```python
from build123d import *

# Parameters (mm, degrees)
SKETCH_1_W           = 58
SKETCH_1_H           = 13
EXTRUDE_1_DEPTH      = 6
SKETCH_9_W           = 58
SKETCH_9_H           = 2.7
EXTRUDE_5_DEPTH      = 22
SKETCH_10_R          = 1.75
CUT_EXTRUDE_6_DEPTH  = 42.606369705
SKETCH_11_W          = 40
SKETCH_11_H          = 20
CUT_EXTRUDE_7_DEPTH  = 42.606369705
SKETCH_13_W          = 2
SKETCH_13_H          = 13
CUT_EXTRUDE_8_DEPTH  = 41.831972766
SKETCH_3_R           = 1.3
SKETCH_3_R_2         = 1.5
CUT_EXTRUDE_9_DEPTH  = 10
SKETCH_14_W          = 40
SKETCH_14_H          = 20
EXTRUDE_6_DEPTH      = 5
SKETCH_15_R          = 1.75
CUT_EXTRUDE_10_DEPTH = 42.606369705
SKETCH_16_W          = 40
SKETCH_16_H          = 1
CUT_EXTRUDE_11_DEPTH = 10
SKETCH_17_W          = 2
SKETCH_17_H          = 21
CUT_EXTRUDE_13_DEPTH = 10
SKETCH_18_W          = 7
SKETCH_18_H          = 1
CUT_EXTRUDE_14_DEPTH = 1.5
FILLET_1_R           = 0.5
SKETCH_21_R          = 1.5
CUT_EXTRUDE_16_DEPTH = 10
FILLET_4_R           = 0.5
SKETCH_23_W          = 7
SKETCH_23_H          = 7.7
EXTRUDE_7_DEPTH      = 3


with BuildPart() as part:
    # 草图1 → 凸台-拉伸1 (new body)
    with BuildSketch(Plane.XY):
        Rectangle(SKETCH_1_W, SKETCH_1_H)
    extrude(amount=EXTRUDE_1_DEPTH)

    # 草图9 → 凸台-拉伸5 (add)
    with BuildSketch(Plane.XY.offset(6)):
        with Locations((0, -5.15)):
            Rectangle(SKETCH_9_W, SKETCH_9_H)
    extrude(amount=EXTRUDE_5_DEPTH)

    # 草图10 → 切除-拉伸6 (cut, through all)
    with BuildSketch(Plane(origin=(0, -3.8, 0), x_dir=(1, 0, 0), z_dir=(0, 1, 0))):
        with Locations(Location((-24.5, -24, 0), (0, 0, 270))):
            Circle(SKETCH_10_R)
        with Locations(Location((-24.5, -14.5, 0), (0, 0, 270))):
            Circle(SKETCH_10_R)
        with Locations(Location((24.5, -24, 0), (0, 0, 270))):
            Circle(SKETCH_10_R)
        with Locations(Location((24.5, -14.5, 0), (0, 0, 270))):
            Circle(SKETCH_10_R)
    extrude(amount=-CUT_EXTRUDE_6_DEPTH, mode=Mode.SUBTRACT)

    # 草图11 → 切除-拉伸7 (cut, through all)
    with BuildSketch(Plane(origin=(0, -3.8, 0), x_dir=(1, 0, 0), z_dir=(0, 1, 0))):
        with Locations((0, -17)):
            Rectangle(SKETCH_11_W, SKETCH_11_H)
    extrude(amount=-CUT_EXTRUDE_7_DEPTH, mode=Mode.SUBTRACT)

    # 草图13 → 切除-拉伸8 (cut, through all)
    with BuildSketch(Plane.XY.offset(28)):
        with Locations((-28, 0)):
            Rectangle(SKETCH_13_W, SKETCH_13_H)
    extrude(amount=-CUT_EXTRUDE_8_DEPTH, mode=Mode.SUBTRACT)

    # 草图3 → 切除-拉伸9 (cut)
    with BuildSketch(Plane(origin=(0, 0, 0), x_dir=(-1, 0, 0), z_dir=(0, 0, -1))):
        with Locations((20, -2.2)):
            Circle(SKETCH_3_R)
        with Locations((9, -0.2)):
            Circle(SKETCH_3_R_2)
    extrude(amount=-CUT_EXTRUDE_9_DEPTH, mode=Mode.SUBTRACT)

    # 草图14 → 凸台-拉伸6 (add)
    with BuildSketch(Plane.XZ.offset(6.5)):
        Polygon((-27, 28), (-20, 28), (20, 28), (29, 28), (29, 0), (-20, 0), (-27, 0), align=None)
        with Locations((0, 17)):
            Rectangle(SKETCH_14_W, SKETCH_14_H, mode=Mode.SUBTRACT)
    extrude(amount=EXTRUDE_6_DEPTH)

    # 草图15 → 切除-拉伸10 (cut, through all)
    with BuildSketch(Plane(origin=(0, -3.8, 0), x_dir=(1, 0, 0), z_dir=(0, 1, 0))):
        with Locations(Location((-24.5, -14.5, 0), (0, 0, 270))):
            Circle(SKETCH_15_R)
        with Locations(Location((-24.5, -24, 0), (0, 0, 270))):
            Circle(SKETCH_15_R)
        with Locations(Location((24.5, -14.5, 0), (0, 0, 270))):
            Circle(SKETCH_15_R)
        with Locations(Location((24.5, -24, 0), (0, 0, 270))):
            Circle(SKETCH_15_R)
    extrude(amount=-CUT_EXTRUDE_10_DEPTH, mode=Mode.SUBTRACT)

    # 草图16 → 切除-拉伸11 (cut)
    with BuildSketch(Plane(origin=(0, -3.8, 0), x_dir=(1, 0, 0), z_dir=(0, 1, 0))):
        with Locations((0, -27.5)):
            Rectangle(SKETCH_16_W, SKETCH_16_H)
    extrude(amount=-CUT_EXTRUDE_11_DEPTH, mode=Mode.SUBTRACT)

    # 草图17 → 切除-拉伸13 (cut)
    with BuildSketch(Plane(origin=(0, -3.8, 0), x_dir=(1, 0, 0), z_dir=(0, 1, 0))):
        with Locations((21, -17.5)):
            Rectangle(SKETCH_17_W, SKETCH_17_H)
    extrude(amount=-CUT_EXTRUDE_13_DEPTH, mode=Mode.SUBTRACT)

    # 草图18 → 切除-拉伸14 (cut)
    with BuildSketch(Plane(origin=(0, -3.8, 0), x_dir=(1, 0, 0), z_dir=(0, 1, 0))):
        with Locations((-23.5, -19.25)):
            Rectangle(SKETCH_18_W, SKETCH_18_H)
        with Locations((25.5, -19.25)):
            Rectangle(SKETCH_18_W, SKETCH_18_H)
    extrude(amount=-CUT_EXTRUDE_14_DEPTH, mode=Mode.SUBTRACT)

    # 圆角1
    fillet_1_edges = [part.edges().sort_by_distance(p)[0] for p in [
        (1, -3.8, 6),
    ]]
    fillet(fillet_1_edges, radius=FILLET_1_R)

    # 草图21 → 切除-拉伸16 (cut)
    with BuildSketch(Plane.XY.offset(6)):
        with Locations((-16, 2.2)):
            Circle(SKETCH_21_R)
    extrude(amount=-CUT_EXTRUDE_16_DEPTH, mode=Mode.SUBTRACT)

    # 圆角4
    fillet_4_edges = [part.edges().sort_by_distance(p)[0] for p in [
        (25.5, -5.3, 19.75),
        (25.5, -5.3, 18.75),
        (-23.5, -5.3, 19.75),
        (-23.5, -5.3, 18.75),
    ]]
    fillet(fillet_4_edges, radius=FILLET_4_R - 0.0001)  # a hair under: the kernel refuses the full size

    # 草图23 → 凸台-拉伸7 (add)
    with BuildSketch(Plane.XY.offset(28)):
        with Locations((-23.5, -7.65)):
            Rectangle(SKETCH_23_W, SKETCH_23_H)
        with Locations((25.5, -7.65)):
            Rectangle(SKETCH_23_W, SKETCH_23_H)
    extrude(amount=EXTRUDE_7_DEPTH)


solid = part.part
```
Verification items for the finished model (mm, model axes). A direction names the side the tool comes from. Give positions to 0.01 mm unless a question says otherwise; leave off trailing zeros. Order: outer loops, then holes, each group sorted by start corner. A loop starts at its lowest first (then second) coordinate and runs counter-clockwise, first axis right, second up. Notation, with made-up numbers: M 54.25,-33.5 L 74.25,-33.5 A21 cw 74.25,-15.5 Z; hole C -14.75,-2.5 d5. An arc over 180 degrees is marked long. Answer in a Markdown table with one row per item. Add a question column.
Item 1: Tool access check on faces 5 (the flat face through (26.2, -3.8, 25.3)), 6 (the cylindrical face through (-18.7, -2.14, 2.96)), 7 (the flat face through (1, -8, 7)), 8 (the flat face through (-24, -4, 18.75)). Record the directions out of +Z, -Z, +X, -X, +Y, -Y that give a thin tool (end or side, any length) a straight path to the whole face; none if there is none.
Item 2: Scan lines: probe 1 along X at (y, z) = (-7, 14.5); probe 2 along Y at (x, z) = (-9, 3.35); probe 3 along X at (y, z) = (-2.2, 3). Record each from-to range of solid material in increasing order. Write a range as from..to.
Item 3: Gauge pin test, flat ends, axial feed: pin 1 (5.5 mm diameter, centred on x = -24.5, z = 23.5, fed in from +Y); pin 2 (3 mm diameter, centred on x = 16, y = 2, fed in from +Z); pin 3 (5 mm diameter, centred on x = -15.5, z = 7.5, fed in from +Y); pin 4 (8 mm diameter, centred on x = 2, y = -3.5, fed in from +Z). Record the tip position at first contact, or that the pin passes through.
Item 4: Section check C-C, the plane y = 2.2. Enter the section's corners in (x, z).
Item 5: Section check D-D, the plane y = -6. Enter the section's corners in (x, z).
Item 6: Section check B-B, the plane z = 14.5. Enter the section's corners in (x, y), and give its area (3 significant figures).
Item 7: Section check A-A, the plane x = -24.5. State how many separate pieces and enclosed holes the cut face has, and give its area (3 significant figures).
Item 8: Mould release check, pull along Z, two halves, no side actions. Record for faces 1 (the cylindrical face through (-22.765, -7.596, 14.272)), 2 (the flat face through (1, -2, 0)), 3 (the flat face through (-22.8, -3.8, 25.3)), 4 (the flat face through (-24, -8, 31)): released by +Z, released by -Z, zero draft, split by the parting line, or undercut.
Filled sheet:
| question | item | result |
|---|---|---|
| 1 | face 5 | +Z, +X, -X, +Y |
| 1 | face 6 | +Z, -Z |
| 1 | face 7 | +Z, +Y, -Y |
| 1 | face 8 | +X, -X, +Y |
| 2 | probe 1 | x = -27..-26.25, -22.75..-20, 22..22.75, 26.25..29 |
| 2 | probe 2 | y = -11.5..-1.7, 1.3..6.5 |
| 2 | probe 3 | x = -27..-21.3, -18.7..29 |
| 3 | pin 1 | stops at y = -3.8 |
| 3 | pin 2 | stops at z = 6 |
| 3 | pin 3 | stops at y = 6.5 |
| 3 | pin 4 | stops at z = 7 |
| 4 | outline | M -27,0 L -17.5,0 L -17.5,6 L -27,6 Z; M -14.5,0 L 29,0 L 29,6 L -14.5,6 Z |
| 5 | outline | M -27,0 L 29,0 L 29,31 L 22,31 L 22,7 L -20,7 L -20,31 L -27,31 Z; hole C -24.5,14.5 d3.5; hole C -24.5,24 d3.5; hole C 24.5,14.5 d3.5; hole C 24.5,24 d3.5 |
| 6 | outline | M -27,-11.5 L -26.25,-11.5 L -26.25,-3.8 L -27,-3.8 Z; M -22.75,-11.5 L -20,-11.5 L -20,-3.8 L -22.75,-3.8 Z; M 22,-11.5 L 22.75,-11.5 L 22.75,-3.8 L 22,-3.8 Z; M 26.25,-11.5 L 29,-11.5 L 29,-3.8 L 26.25,-3.8 Z |
| 6 | area | 53.9 mm^2 |
| 7 | separate pieces | 3 |
| 7 | enclosed holes | 0 |
| 7 | area | 245 mm^2 |
| 8 | face 1 | undercut |
| 8 | face 2 | released by -Z |
| 8 | face 3 | zero draft |
| 8 | face 4 | released by +Z |
